```python
from build123d import *

# Parameters (mm, degrees)
SKETCH1_R           = 2.6
BOSS_EXTRUDE1_DEPTH = 20
BOSS_EXTRUDE2_DEPTH = 20


with BuildPart() as part:
    # Sketch1 → Boss-Extrude1 (new body)
    with BuildSketch(Plane(origin=(0, 0, 0), x_dir=(1, 0, 0), z_dir=(0, 1, 0))):
        with BuildLine():
            Line((10, 0), (-10, 0))
            ThreePointArc((-10, 0), (-2.947752983, 31.810630591), (16.887506811, 57.660444431))
            Line((16.887506811, 57.660444431), (29.743259005, 42.339555569))
            ThreePointArc((29.743259005, 42.339555569), (15.178402758, 23.358265357), (10, 0))
        make_face()
        with Locations(Location((0.770593323, 10, 0), (0, 0, 270))):
            Circle(SKETCH1_R, mode=Mode.SUBTRACT)
        with Locations(Location((6.115324888, 27.584447974, 0), (0, 0, 270))):
            Circle(SKETCH1_R, mode=Mode.SUBTRACT)
        with Locations(Location((16.150266317, 42.98181517, 0), (0, 0, 270))):
            Circle(SKETCH1_R, mode=Mode.SUBTRACT)
    extrude(amount=BOSS_EXTRUDE1_DEPTH)

    # Sketch2 → Boss-Extrude2 (add)
    with BuildSketch(Plane(origin=(0, 20, 0), x_dir=(1, 0, 0), z_dir=(0, 1, 0))):
        Polygon((16.887506811, 57.660444431), (29.743259005, 42.339555569), (34.416130108, 46.260559988), (21.560377914, 61.58144885), align=None)
    extrude(amount=-BOSS_EXTRUDE2_DEPTH)


solid = part.part
```
The model under review builds one solid part; all positions refer to its coordinate system, in mm. Round coordinates to 2 decimals unless told otherwise and drop trailing zeros. Order: outer loops, then holes, each group sorted by start corner. A loop starts at its lowest first (then second) coordinate and runs counter-clockwise, first axis right, second up. Notation, with made-up numbers: M 1,49 L 37,49 A15 ccw 37,55 Z; hole C 85.5,47.25 d6. An arc over 180 degrees is marked long. Use a Markdown table: item, result.
1) Consider section D-D (x = 29). Write out the cut boundary in (y, z).
Report:
| item | result |
|---|---|
| outline | M 0,-52.72 L 20,-52.72 L 20,-41.7 L 0,-41.7 Z |
2) Draft analysis for pull direction Z (two halves, no side actions). For faces 1 (the face through (7, 0, -31)), 2 (the face through (6.896, 9.86, -25.105)), 3 (the face through (28.08, 10.14, -53.81)), 4 (the face through (0, 10, 0)), state which applies: released by +Z, released by -Z, zero draft, split by the parting line, or undercut.
Report:
| item | result |
|---|---|
| face 1 | zero draft |
| face 2 | undercut |
| face 3 | released by -Z |
| face 4 | released by +Z |
3) Consider section C-C (y = 9). Write out the cut boundary in (x, z).
Report:
| item | result |
|---|---|
| outline | M -10,0 A75.27 ccw 16.89,-57.66 L 21.56,-61.58 L 34.42,-46.26 L 29.74,-42.34 A55.27 cw 10,0 Z; hole C 0.77,-10 d5.2; hole C 6.12,-27.58 d5.2; hole C 16.15,-42.98 d5.2 |
4) Consider section B-B (x = 2). Write out the cut boundary in (y, z), then the cut area to 3 significant figures.
Report:
| item | result |
|---|---|
| outline | M 0,-40.77 L 20,-40.77 L 20,-12.29 L 0,-12.29 Z; M 0,-7.71 L 20,-7.71 L 20,0 L 0,0 Z |
| area | 724 mm^2 |
5) Wall thickness on line 1 along Z through (x, y) = (15, 7.5); line 2 along Z through (x, y) = (-1, 18); line 3 along X through (y, z) = (14.75, -42): over which ranges is each line inside the solid? List them lowest first. Write a range as [from, to].
Report:
| item | result |
|---|---|
| line 1 | [-56.02, -45.31], [-40.65, -22.97] |
| line 2 | [-35.69, -11.9], [-8.1, 0] |
| line 3 | [2.81, 13.74], [18.56, 29.34] |
6) Consider section A-A (z = -27.5). Write out the cut boundary in (x, y), then the cut area to 3 significant figures.
Report:
| item | result |
|---|---|
| outline | M -4.8,0 L 3.52,0 L 3.52,20 L -4.8,20 Z; M 8.71,0 L 17.33,0 L 17.33,20 L 8.71,20 Z |
| area | 339 mm^2 |
7) Insertion check: pin 1 (10 mm diameter, centred on x = 26.5, z = -30.5, fed in from -Y); pin 2 (6 mm diameter, centred on x = 24.5, y = 15, fed in from -Z); pin 3 (5 mm diameter, centred on y = 4.5, z = -51.5, fed in from +X); pin 4 (4 mm diameter, centred on y = 15, z = -38, fed in from -X). Each pin has a flat end and moves straight along its axis. Give the tip position at first contact, or say it passes through.
Report:
| item | result |
|---|---|
| pin 1 | through |
| pin 2 | z = -61.58 |
| pin 3 | x = 32.12 |
| pin 4 | x = -0.83 |
